from build123d import *

# Parameters (mm, degrees)
F0_W     = 850
F0_H     = 600
F0_R     = 5.5
F0_R_2   = 4.5
F0_R_3   = 20
F1_DEPTH = 5
F2_R     = 5


with BuildPart() as f1:
    # F0 (on Front) → F1 (new body)
    with BuildSketch(Plane.XZ):
        Rectangle(F0_W, F0_H)
        with Locations((-388, -122.5)):
            Circle(F0_R, mode=Mode.SUBTRACT)
        with Locations((-338, -122.5)):
            Circle(F0_R, mode=Mode.SUBTRACT)
        with Locations((-378, -101.5)):
            Circle(F0_R_2, mode=Mode.SUBTRACT)
        with Locations((-328, -101.5)):
            Circle(F0_R_2, mode=Mode.SUBTRACT)
        with Locations((-278, -101.5)):
            Circle(F0_R_2, mode=Mode.SUBTRACT)
        with Locations((-228, -101.5)):
            Circle(F0_R_2, mode=Mode.SUBTRACT)
        with Locations((-320, -62.5)):
            Circle(F0_R, mode=Mode.SUBTRACT)
        with Locations((-320, -42.5)):
            Circle(F0_R_2, mode=Mode.SUBTRACT)
        with Locations((-270, -62.5)):
            Circle(F0_R, mode=Mode.SUBTRACT)
        with Locations((-270, -42.5)):
            Circle(F0_R_2, mode=Mode.SUBTRACT)
        with Locations((-220, -42.5)):
            Circle(F0_R_2, mode=Mode.SUBTRACT)
        with Locations((-178, -101.5)):
            Circle(F0_R_2, mode=Mode.SUBTRACT)
        with Locations((-170, -42.5)):
            Circle(F0_R_2, mode=Mode.SUBTRACT)
        with Locations((-120, -42.5)):
            Circle(F0_R_2, mode=Mode.SUBTRACT)
        with Locations((178, -101.5)):
            Circle(F0_R_2, mode=Mode.SUBTRACT)
        with Locations((120, -42.5)):
            Circle(F0_R_2, mode=Mode.SUBTRACT)
        with Locations((170, -42.5)):
            Circle(F0_R_2, mode=Mode.SUBTRACT)
        with Locations((228, -101.5)):
            Circle(F0_R_2, mode=Mode.SUBTRACT)
        with Locations((278, -101.5)):
            Circle(F0_R_2, mode=Mode.SUBTRACT)
        with Locations((338, -122.5)):
            Circle(F0_R, mode=Mode.SUBTRACT)
        with Locations((388, -122.5)):
            Circle(F0_R, mode=Mode.SUBTRACT)
        with Locations((328, -101.5)):
            Circle(F0_R_2, mode=Mode.SUBTRACT)
        with Locations((378, -101.5)):
            Circle(F0_R_2, mode=Mode.SUBTRACT)
        with Locations((220, -42.5)):
            Circle(F0_R_2, mode=Mode.SUBTRACT)
        with Locations((270, -62.5)):
            Circle(F0_R, mode=Mode.SUBTRACT)
        with Locations((270, -42.5)):
            Circle(F0_R_2, mode=Mode.SUBTRACT)
        with Locations((320, -62.5)):
            Circle(F0_R, mode=Mode.SUBTRACT)
        with Locations((320, -42.5)):
            Circle(F0_R_2, mode=Mode.SUBTRACT)
        with Locations((-320, 42.5)):
            Circle(F0_R_2, mode=Mode.SUBTRACT)
        with Locations((-320, 62.5)):
            Circle(F0_R, mode=Mode.SUBTRACT)
        with Locations((-270, 42.5)):
            Circle(F0_R_2, mode=Mode.SUBTRACT)
        with Locations((-270, 62.5)):
            Circle(F0_R, mode=Mode.SUBTRACT)
        with Locations((-220, 42.5)):
            Circle(F0_R_2, mode=Mode.SUBTRACT)
        with Locations((-378, 85.5)):
            Circle(F0_R_2, mode=Mode.SUBTRACT)
        with Locations((-328, 85.5)):
            Circle(F0_R_2, mode=Mode.SUBTRACT)
        with Locations((-388, 122.5)):
            Circle(F0_R, mode=Mode.SUBTRACT)
        with Locations((-338, 122.5)):
            Circle(F0_R, mode=Mode.SUBTRACT)
        with Locations((-278, 85.5)):
            Circle(F0_R_2, mode=Mode.SUBTRACT)
        with Locations((-228, 85.5)):
            Circle(F0_R_2, mode=Mode.SUBTRACT)
        with Locations((-170, 42.5)):
            Circle(F0_R_2, mode=Mode.SUBTRACT)
        with Locations((-120, 42.5)):
            Circle(F0_R_2, mode=Mode.SUBTRACT)
        Circle(F0_R_3, mode=Mode.SUBTRACT)
        with Locations((-178, 85.5)):
            Circle(F0_R_2, mode=Mode.SUBTRACT)
        with Locations((120, 42.5)):
            Circle(F0_R_2, mode=Mode.SUBTRACT)
        with Locations((170, 42.5)):
            Circle(F0_R_2, mode=Mode.SUBTRACT)
        with Locations((178, 85.5)):
            Circle(F0_R_2, mode=Mode.SUBTRACT)
        with Locations((220, 42.5)):
            Circle(F0_R_2, mode=Mode.SUBTRACT)
        with Locations((270, 42.5)):
            Circle(F0_R_2, mode=Mode.SUBTRACT)
        with Locations((270, 62.5)):
            Circle(F0_R, mode=Mode.SUBTRACT)
        with Locations((320, 42.5)):
            Circle(F0_R_2, mode=Mode.SUBTRACT)
        with Locations((320, 62.5)):
            Circle(F0_R, mode=Mode.SUBTRACT)
        with Locations((228, 85.5)):
            Circle(F0_R_2, mode=Mode.SUBTRACT)
        with Locations((278, 85.5)):
            Circle(F0_R_2, mode=Mode.SUBTRACT)
        with Locations((328, 85.5)):
            Circle(F0_R_2, mode=Mode.SUBTRACT)
        with Locations((378, 85.5)):
            Circle(F0_R_2, mode=Mode.SUBTRACT)
        with Locations((338, 122.5)):
            Circle(F0_R, mode=Mode.SUBTRACT)
        with Locations((388, 122.5)):
            Circle(F0_R, mode=Mode.SUBTRACT)
    extrude(amount=F1_DEPTH)

    # F2
    f2_edges = [f1.edges().sort_by_distance(p)[0] for p in [
        (-425, -2.5, 300),
        (425, -2.5, 300),
        (425, -2.5, -300),
        (-425, -2.5, -300),
    ]]
    fillet(f2_edges, radius=F2_R)


solid = f1.part
For this review, take the finished solid that the model builds, in its own axes (mm). Coordinates: 2 decimals unless noted, no trailing zeros. Loops run counter-clockwise (first coordinate to the right, second up) from the corner with the lowest first, then second, coordinate; pieces in that order, holes last. Notation, with made-up numbers: (24.5, 62.5) - (63.5, 62.5) arc R16 cw to (63.5, 81.5) - close; hole circle Ø4 at (71, -10.5). An arc over 180 degrees is marked (long way). Use a Markdown table: item, result. Add a question column.
Item 1: For line 1 (Z direction, x = -320, y = -1.45); line 2 (Z direction, x = -179, y = -1.85); line 3 (Z direction, x = -278, y = -2.85), list the stretches that pass through material, from the lowest coordinate up.
Item 2: Mouldability with a two-part tool opening along X and no side actions: class faces 1 (the face through (-6, 0, 71)), 2 (the face through (-4.336, -2.465, -19.524)) as pulls with the +X half, pulls with the -X half, needs draft (parallel to the pull), parting line crosses it, or undercut.
Item 3: We need section A-A (x = 0). Give the boundary of the cut face in (y, z), and give its area (3 significant figures).
Results list:
| question | item | result |
|---|---|---|
| 1 | line 1 | z = -300 to -68, -57 to -47, -38 to 38, 47 to 57, 68 to 300 |
| 1 | line 2 | z = -300 to -105.89, -97.11 to 81.11, 89.89 to 300 |
| 1 | line 3 | z = -300 to -106, -97 to 81, 90 to 300 |
| 2 | face 1 | needs draft |
| 2 | face 2 | undercut |
| 3 | outline | (-5, -300) - (0, -300) - (0, -20) - (-5, -20) - close; (-5, 20) - (0, 20) - (0, 300) - (-5, 300) - close |
| 3 | area | 2,800 mm^2 |
